Here's the drawing with two shaded views (mm, measured from the low corner). I have some questions. A direction names the side the tool comes from. Coordinates: 2 decimals unless noted, no trailing zeros. Write each loop counter-clockwise with the first axis right and the second up, starting at its lowest first coordinate (ties: lowest second). Pieces come first, ordered by that corner, then holes. Notation, with made-up numbers: (-25.75, 36) -> (2.25, 36) arc R20 ccw to (2.25, 41) -> close; hole circle Ø10 at (-12.5, -21). An arc over 180 degrees is marked (long way). Answer in a Markdown table with one row per item. Add a question column.
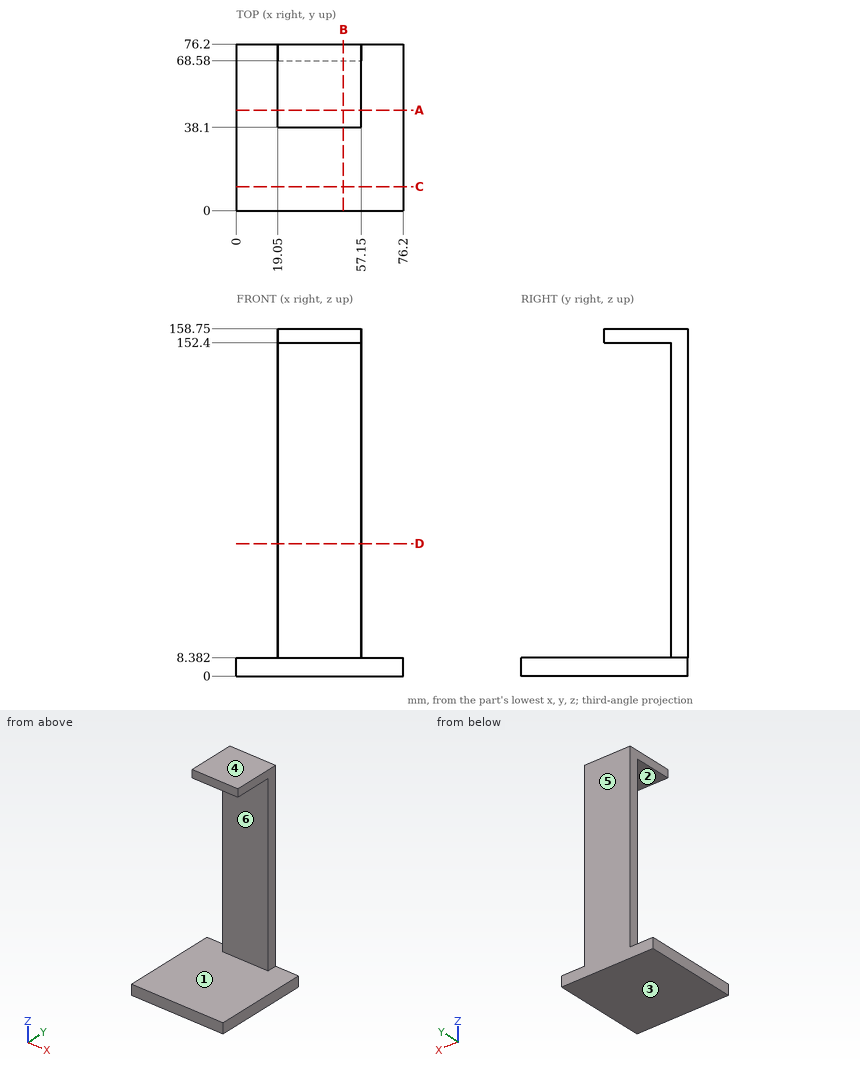
Q1. Imagine slicing it at A-A on y = 46. Please give me the cut outline in (x, z), plus the area to 3 significant figures.
Q2. If we mould it in two halves opening along Z, with no side actions, what happens to the marked faces 1, 2, 3 and 4? For each: pulls with the +Z half, pulls with the -Z half, needs draft (parallel to the pull), parting line crosses it, or undercut.
Q3. Imagine slicing it at B-B on x = 49. Please give me the cut outline in (y, z).
Q4. I'm going to push flat-ended pins straight in: P1, Ø3, axis at x = 28, z = 70.5, coming from the -Y side; P2, Ø7, axis at x = 30.5, z = 157, coming from the -Y side. Where does each tip first touch, or does it pass through?
Q5. I need wall thicknesses on line 1 (Z direction, x = 52, y = 68); line 2 (Y direction, x = 25.5, z = 47.5); line 3 (Z direction, x = 56.5, y = 4). Which ranges of each line are inside material? Lowest first, please. Write a range as [from, to].
Q6. For the marked faces 5 and 6, which set-ups out of +Z, -Z, +X, -X, +Y, -Y let a thin tool reach every point of the face, with its end or its side?
Q7. Imagine slicing it at C-C on y = 11. Please give me the cut outline in (x, z).
Q8. Imagine slicing it at D-D on z = 60.5. Please give me the cut outline in (x, y), plus the area to 3 significant figures.
Result sheet:
| question | item | result |
|---|---|---|
| 1 | outline | (0, 0) -> (76.2, 0) -> (76.2, 8.38) -> (0, 8.38) -> close; (19.05, 152.4) -> (57.15, 152.4) -> (57.15, 158.75) -> (19.05, 158.75) -> close |
| 1 | area | 881 mm^2 |
| 2 | face 1 | undercut |
| 2 | face 2 | undercut |
| 2 | face 3 | pulls with the -Z half |
| 2 | face 4 | pulls with the +Z half |
| 3 | outline | (0, 0) -> (76.2, 0) -> (76.2, 158.75) -> (38.1, 158.75) -> (38.1, 152.4) -> (68.58, 152.4) -> (68.58, 8.38) -> (0, 8.38) -> close |
| 4 | P1 | stops at y = 68.58 |
| 4 | P2 | stops at y = 38.1 |
| 5 | line 1 | z = [0, 8.38], [152.4, 158.75] |
| 5 | line 2 | y = [68.58, 76.2] |
| 5 | line 3 | z = [0, 8.38] |
| 6 | face 5 | +Z, -Z, +X, -X, +Y |
| 6 | face 6 | +X, -X, -Y |
| 7 | outline | (0, 0) -> (76.2, 0) -> (76.2, 8.38) -> (0, 8.38) -> close |
| 8 | outline | (19.05, 68.58) -> (57.15, 68.58) -> (57.15, 76.2) -> (19.05, 76.2) -> close |
| 8 | area | 290 mm^2 |
